Design review of the part built by this model. Coordinates are the model's own, in mm. Face numbers are marked on the shaded views. A direction names the side the tool comes from. Coordinates: 2 decimals unless noted, no trailing zeros. Loops run counter-clockwise (first coordinate to the right, second up) from the corner with the lowest first, then second, coordinate; pieces in that order, holes last. Notation, with made-up numbers: M 30.5,80.25 L 57.5,80.25 A28 cw 57.5,110.25 Z; hole C 28,-7.75 d2. An arc over 180 degrees is marked long. One line per item, written item: value.
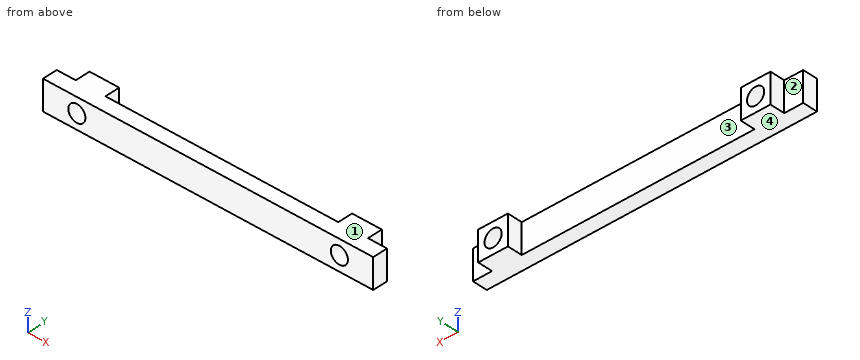
```python
from build123d import *

# Parameters (mm, degrees)
SKETCH1_W             = 6.35
SKETCH1_H             = 3.175
BOSS_EXTRUDE1_DEPTH   = 6.35
F_6_CLEARANCE_HOLE1_D = 3.6576


with BuildPart() as part:
    # Sketch1 → Boss-Extrude1 (new body)
    with BuildSketch(Plane.XY):
        Polygon((0, 0), (35.306, 0), (35.306, 3.175), (10.414, 3.175), (4.064, 3.175), (0, 3.175), align=None)
        with Locations((7.239, 4.7625)):
            Rectangle(SKETCH1_W, SKETCH1_H)
        with Locations((63.373, 4.7625)):
            Rectangle(SKETCH1_W, SKETCH1_H)
        Polygon((35.306, 3.175), (35.306, 0), (70.612, 0), (70.612, 3.175), (66.548, 3.175), (60.198, 3.175), align=None)
    extrude(amount=BOSS_EXTRUDE1_DEPTH)

    # #6 Clearance Hole1 (through all)
    with Locations(Plane(origin=(7.239, 0, 3.175), x_dir=(0, 0, -1), z_dir=(0, -1, 0))):
        with Locations((0, 0), (0, 56.134)):
            Hole(F_6_CLEARANCE_HOLE1_D / 2)


solid = part.part
```
(1) We need section A-A on y = 5.75. State the section outline as (x, z) points (3 decimals), then the cut area to 3 significant figures.
Reply:
outline: M 4.064,0 L 10.414,0 L 10.414,6.35 L 4.064,6.35 Z; M 60.198,0 L 66.548,0 L 66.548,6.35 L 60.198,6.35 Z; hole C 7.239,3.175 d3.658; hole C 63.373,3.175 d3.658
area: 59.6 mm2
(2) We need section C-C on z = 3.5. State the section outline as (x, y) points (3 decimals), then the cut area to 3 significant figures.
Reply:
outline: M 0,0 L 5.439,0 L 5.439,6.35 L 4.064,6.35 L 4.064,3.175 L 0,3.175 Z; M 9.039,0 L 61.573,0 L 61.573,6.35 L 60.198,6.35 L 60.198,3.175 L 10.414,3.175 L 10.414,6.35 L 9.039,6.35 Z; M 65.173,0 L 70.612,0 L 70.612,3.175 L 66.548,3.175 L 66.548,6.35 L 65.173,6.35 Z
area: 219 mm2
(3) Insertion check: pin 1 (1.2 mm diameter, centred on x = 3, z = 3, fed in from +Y) (3 decimals); pin 2 (1.6 mm diameter, centred on y = 4.5, z = 3, fed in from -X); pin 3 (3.5 mm diameter, centred on y = 4.5, z = 4.5, fed in from +X); pin 4 (2.5 mm diameter, centred on y = 5.5, z = 3.5, fed in from +X). Each pin has a flat end and moves straight along its axis. Give the tip position at first contact, or say it passes through.
Reply:
pin 1: stops at y = 3.175
pin 2: stops at x = 4.06
pin 3: stops at x = 70.61
pin 4: stops at x = 66.55
(4) We need section B-B on x = 6.5. State the section outline as (y, z) points.
Reply:
outline: M 0,0 L 6.35,0 L 6.35,1.5 L 0,1.5 Z; M 0,4.85 L 6.35,4.85 L 6.35,6.35 L 0,6.35 Z
(5) To check wall thickness, follow line 1 along X through (y, z) = (2.5, 3.25); line 2 along X through (y, z) = (1, 1.5); line 3 along X through (y, z) = (6, 1.5). State the ranges of each line that lie inside material, in increasing order. Write a range as [from, to].
Reply:
line 1: x = [0, 5.41], [9.07, 61.55], [65.2, 70.61]
line 2: x = [0, 6.5], [7.97, 62.64], [64.11, 70.61]
line 3: x = [4.06, 6.5], [7.97, 10.41], [60.2, 62.64], [64.11, 66.55]
(6) We need section D-D on x = 20. State the section outline as (y, z) points (3 decimals).
Reply:
outline: M 0,0 L 3.175,0 L 3.175,6.35 L 0,6.35 Z
(7) Tool access review of the marked faces 1 and 2: name each direction out of +Z, -Z, +X, -X, +Y, -Y from which nothing blocks a thin tool from reaching the whole face with its end or side.
Reply:
face 1: +Z, +X, -X, +Y, -Y
face 2: +Z, -Z, -X, +Y
(8) Mouldability with a two-part tool opening along X and no side actions: class the marked faces 3 and 4 as released by +X, released by -X, zero draft, split by the parting line, or undercut.
Reply:
face 3: undercut
face 4: zero draft
